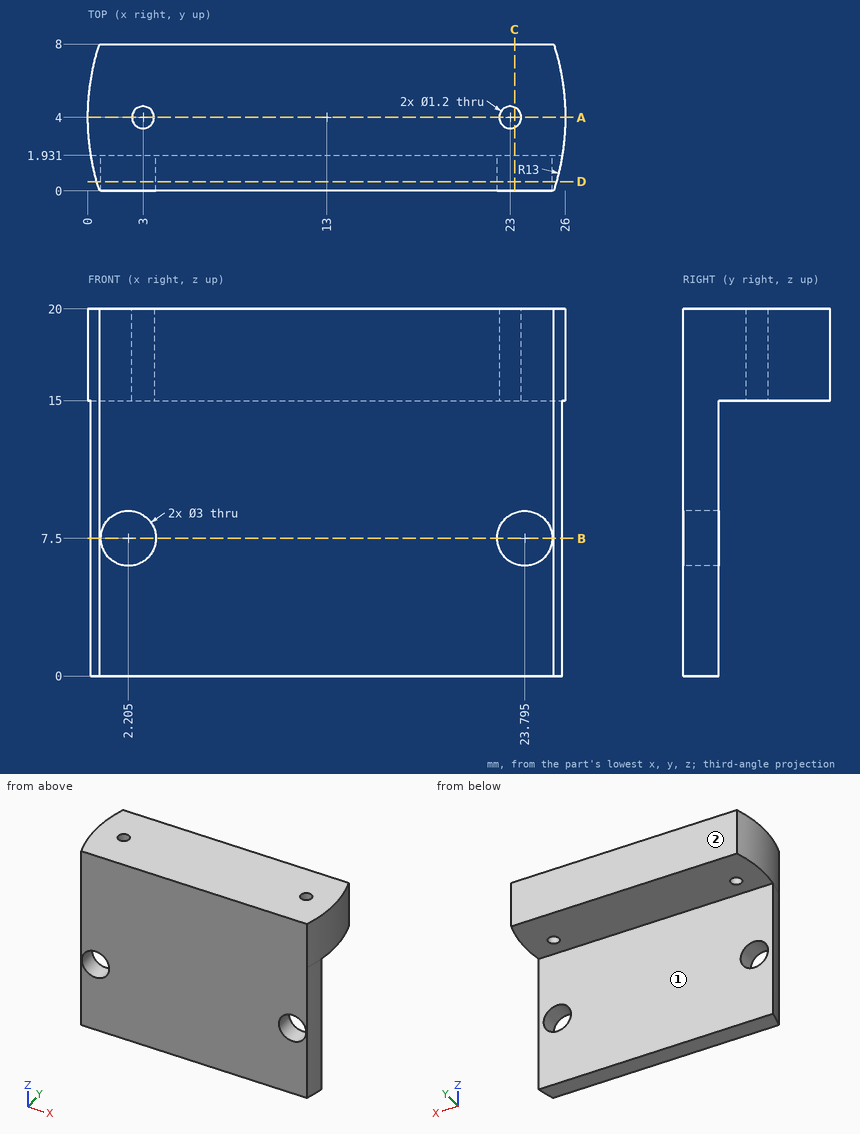
Here's the drawing with two shaded views (mm, measured from the low corner). I have some questions. A direction names the side the tool comes from. Coordinates: 2 decimals unless noted, no trailing zeros. Loops run counter-clockwise (first coordinate to the right, second up) from the corner with the lowest first, then second, coordinate; pieces in that order, holes last. Notation, with made-up numbers: M -34.75,65 L -30.75,65 A27 ccw -30.75,85 Z; hole C 43.25,72 d10. An arc over 180 degrees is marked long. Return JSON: item names as keys, results as strings. Group by question number.
Item 1: Imagine slicing it at C-C (x = 23.25). Please give me the cut outline in (y, z).
Item 2: Imagine slicing it at A-A (y = 4). Please give me the cut outline in (x, z).
Item 3: I'm going to push flat-ended pins straight in: pin 1 Ø1.8 at (x, z) = (23.795, 7.5) entering from -Y; pin 2 Ø2 at (x, z) = (13, 4) entering from +Y; pin 3 Ø2 at (x, y) = (8.5, 3) entering from -Z. Where does each tip first touch, or does it pass through?
Item 4: Imagine slicing it at D-D (y = 0.5). Please give me the cut outline in (x, z) (3 decimals), and give its area (3 significant figures).
Item 5: On a 3-axis mill with a long thin cutter (end or side, diameter ignored), from which of +Z, -Z, +X, -X, +Y, -Y can I reach the whole of each face in a straight line? I mean the marked faces 1 and 2. Say none if no direction works.
Item 6: If I drill on L1, parallel to Y at x = 23, z = 18.05; L2, parallel to X at y = 0.8, z = 7.5 (3 decimals); L3, parallel to Z at x = 15, y = 3, over which ranges is the centre line in solid material (lowest first)? Write a range as from..to.
Item 7: Imagine slicing it at B-B (z = 7.5). Please give me the cut outline in (x, y) (3 decimals).
Verdict:
{
 "1": {"outline": "M 0,0 L 1.93,0 L 1.93,6.1 L 0,6.1 Z; M 0,8.9 L 1.93,8.9 L 1.93,15 L 3.45,15 L 3.45,20 L 0,20 Z; M 4.55,15 L 8,15 L 8,20 L 4.55,20 Z"},
 "2": {"outline": "M 0,15 L 2.4,15 L 2.4,20 L 0,20 Z; M 3.6,15 L 22.4,15 L 22.4,20 L 3.6,20 Z; M 23.6,15 L 26,15 L 26,20 L 23.6,20 Z"},
 "3": {"pin 1": "passes through", "pin 2": "stops at y = 1.93", "pin 3": "stops at z = 15"},
 "4": {"outline": "M 0.48,0 L 25.52,0 L 25.52,20 L 0.48,20 Z; hole C 2.205,7.5 d3; hole C 23.795,7.5 d3", "area": "487 mm^2"},
 "5": {"face 1": "-Z, +X, -X, +Y", "face 2": "+Z, -Z, +X, -X, +Y"},
 "6": {"L1": "y = 0..3.4, 4.6..8", "L2": "x = 0.4..0.705, 3.705..22.295, 25.295..25.6", "L3": "z = 15..20"},
 "7": {"outline": "M 0.166,1.931 A13 ccw 0.631,0 L 0.705,0 L 0.705,1.931 Z; M 3.705,0 L 22.295,0 L 22.295,1.931 L 3.705,1.931 Z; M 25.295,0 L 25.369,0 A13 ccw 25.834,1.931 L 25.295,1.931 Z"}
}
